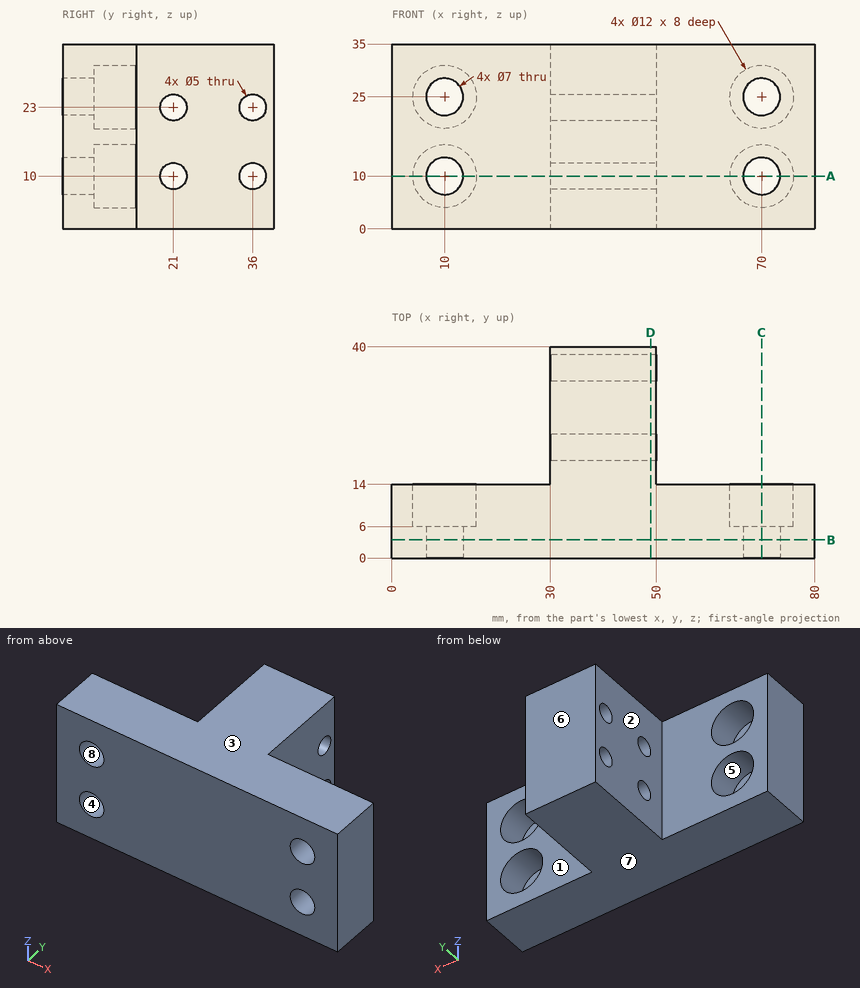
Study the drawing (mm; zero at the part's minimum x, y, z) and answer. A direction names the side the tool comes from. Give positions to 0.01 mm unless a question says otherwise; leave off trailing zeros. Order: outer loops, then holes, each group sorted by start corner. A loop starts at its lowest first (then second) coordinate and runs counter-clockwise, first axis right, second up.
1) Find section C-C on x = 70. Write down the section's boundary in (y, z), then the cut area to 3 significant figures.
Reported:
outline: (0, 0) - (14, 0) - (14, 4) - (6, 4) - (6, 6.5) - (0, 6.5) - close; (0, 13.5) - (6, 13.5) - (6, 16) - (14, 16) - (14, 19) - (6, 19) - (6, 21.5) - (0, 21.5) - close; (0, 28.5) - (6, 28.5) - (6, 31) - (14, 31) - (14, 35) - (0, 35) - close
area: 214 mm2
2) Given P1, Ø9, axis at x = 10, z = 25, coming from the +Y side; P2, Ø9.5, axis at x = 71.5, z = 24.5, coming from the +Y side; P3, Ø6.5, axis at x = 70, z = 10, coming from the -Y side; P4, Ø13, axis at y = 31.5, z = 20, coming from the +X side, each flat-ended and moving along its own axis, determine where each tip first touches the part or whether it passes through.
Reported:
P1: stops at y = 6
P2: stops at y = 14
P3: passes through
P4: stops at x = 50
3) For the marked faces 1, 2, 3, 4 and 5, determine the directions among +Z, -Z, +X, -X, +Y, -Y from which every point of the face is accessible in a straight line to the end or side of a thin tool.
Reported:
face 1: +Z, -Z, +X, +Y
face 2: +Z, -Z, -X, +Y
face 3: +Z, +X, -X, +Y, -Y
face 4: +Y, -Y
face 5: +Y
4) Determine the mould class of the marked faces 6, 7 and 8 for opening direction Z: pulls with the +Z half, pulls with the -Z half, needs draft (parallel to the pull), parting line crosses it, or undercut.
Reported:
face 6: needs draft
face 7: pulls with the -Z half
face 8: undercut
5) Find section D-D on x = 49. Write down the section's boundary in (y, z), then the cut area to 3 significant figures.
Reported:
outline: (0, 0) - (40, 0) - (40, 35) - (0, 35) - close; hole circle Ø5 at (21, 10); hole circle Ø5 at (21, 23); hole circle Ø5 at (36, 10); hole circle Ø5 at (36, 23)
area: 1,320 mm2
6) Find section A-A on z = 10. Give the number of separate pieces and of enclosed holes in the cut face, then the cut area to 3 significant figures.
Reported:
separate pieces: 5
enclosed holes: 0
area: 1,160 mm2
7) Find section B-B on y = 3.5. Write down the section's boundary in (x, z), then the cut area to 3 significant figures.
Reported:
outline: (0, 0) - (80, 0) - (80, 35) - (0, 35) - close; hole circle Ø7 at (10, 10); hole circle Ø7 at (10, 25); hole circle Ø7 at (70, 10); hole circle Ø7 at (70, 25)
area: 2,650 mm2
8) Consider line 1 along Y through (x, z) = (34, 10); line 2 along X through (y, z) = (3, 25); line 3 along Z through (x, y) = (10, 2.3). Determine where each line is inside the solid, lowest interval first.
Reported:
line 1: y = 0 to 18.5, 23.5 to 33.5, 38.5 to 40
line 2: x = 0 to 6.5, 13.5 to 66.5, 73.5 to 80
line 3: z = 0 to 6.5, 13.5 to 21.5, 28.5 to 35
